```python
from build123d import *

# Parameters (mm, degrees)
BOSS_EXTRUDE1_DEPTH = 4.45


with BuildPart() as part:
    # Sketch1 → Boss-Extrude1 (new body)
    with BuildSketch(Plane.XY):
        with BuildLine():
            Line((-1.5, 0), (-1.5, -2))
            ThreePointArc((-1.5, -2), (0, 2.5), (1.5, -2))
            Line((1.5, -2), (1.5, 0))
            ThreePointArc((1.5, 0), (0, 1.5), (-1.5, 0))
        make_face()
    extrude(amount=BOSS_EXTRUDE1_DEPTH)

    # Sketch3 → Revolve3 (revolve)
    with BuildSketch(Plane(origin=(0, 0, 0), x_dir=(0, 0, -1), z_dir=(1, 0, 0))):
        with BuildLine():
            Line((0, 2.5), (0.177867067, 3.270426908))
            Line((0.177867067, 3.270426908), (-0.06572545, 3.326664671))
            Line((-0.06572545, 3.326664671), (0.254829803, 4.715142014))
            ThreePointArc((0.254829803, 4.715142014), (0.404744943, 4.80881939), (0.311067566, 4.95873453))
            Line((0.311067566, 4.95873453), (1.149010244, 8.588263021))
            Line((1.149010244, 8.588263021), (0.087181853, 8.833405421))
            Line((0.087181853, 8.833405421), (-1.496634638, 1.973142501))
            Line((-1.496634638, 1.973142501), (-0.191213731, 1.671762337))
            Line((-0.191213731, 1.671762337), (0, 2.5))
        make_face()
    revolve(axis=Axis((0, 8.833405421, -0.087181853), (0, -0.974370065, 0.224951054)))


solid = part.part
```
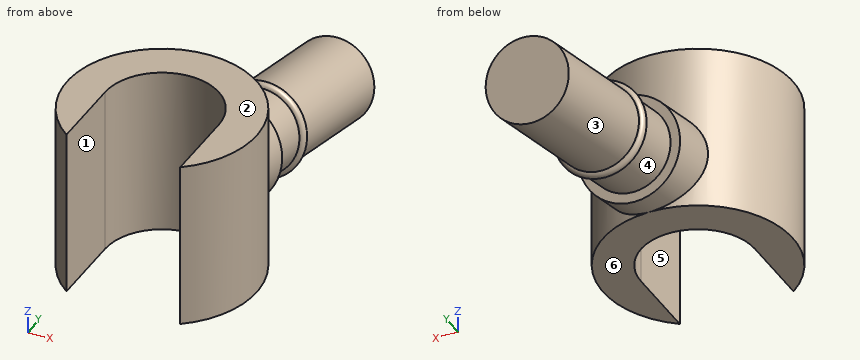
For this review, take the finished solid that the model builds, in its own axes (mm). Face numbers are marked on the shaded views. A direction names the side the tool comes from. Coordinates: 2 decimals unless noted, no trailing zeros. Loops run counter-clockwise (first coordinate to the right, second up) from the corner with the lowest first, then second, coordinate; pieces in that order, holes last. Notation, with made-up numbers: (87.5, -37.5) -> (128.5, -37.5) arc R28 cw to (128.5, -7.5) -> close; hole circle Ø6 at (-8.75, 6). An arc over 180 degrees is marked (long way). Return JSON: item names as keys, results as strings. Group by question number.
(1) To check wall thickness, follow L1, parallel to Z at x = 2, y = -0.5; L2, parallel to Y at x = 2.25, z = 1; L3, parallel to X at y = 0.75, z = 3.3. State the ranges of each line that lie inside material, in increasing order.
(2) Consider section A-A, the plane z = 3.45. Give the boundary of the cut face in (x, y).
(3) Mouldability with a two-part tool opening along X and no side actions: class the marked faces 1, 2 and 3 as pulls with the +X half, pulls with the -X half, needs draft (parallel to the pull), parting line crosses it, or undercut.
(4) Tool access review of the marked faces 4, 5 and 6: name each direction out of +Z, -Z, +X, -X, +Y, -Y from which nothing blocks a thin tool from reaching the whole face with its end or side.
(5) Consider section B-B, the plane x = 2. Give the boundary of the cut face in (y, z), plus the area to 4 significant figures.
(6) For pin 1 Ø3 at (x, y) = (0, 0.5) entering from -Z; pin 2 Ø0.6 at (y, z) = (-1, 2.5) entering from +X; pin 3 Ø1 at (y, z) = (-1, 1.5) entering from -X, all flat-tipped, find the tip position at first contact; note any pin that passes through.
Results below:
{
 "1": {"L1": "z = 0 to 4.45", "L2": "y = -1.09 to 1.09", "L3": "x = -2.38 to -1.3, 1.3 to 2.38"},
 "2": {"outline": "(-1.5, -2) -> (-1.5, 0) arc R1.5 cw to (1.5, 0) -> (1.5, -2) arc R2.5 ccw (long way) to start"},
 "3": {"face 1": "undercut", "face 2": "needs draft", "face 3": "parting line crosses it"},
 "4": {"face 4": "none", "face 5": "+Z, -Z, -Y", "face 6": "-Z, +X, -X, -Y"},
 "5": {"outline": "(-1.5, 0) -> (1.5, 0) -> (1.5, 4.45) -> (-1.5, 4.45) -> close", "area": "13.35 mm2"},
 "6": {"pin 1": "stops at z = 0", "pin 2": "stops at x = 2.4", "pin 3": "stops at x = -2.45"}
}
